from build123d import *

# Parameters (mm, degrees)
CROQUIS2_R              = 5.5
SALIENTE_EXTRUIR1_DEPTH = 18
SALIENTE_EXTRUIR2_DEPTH = 6
CROQUIS4_R              = 3
CORTAR_EXTRUIR1_DEPTH   = 12
CROQUIS5_R              = 1.5
CORTAR_EXTRUIR2_DEPTH   = 6


with BuildPart() as part:
    # Croquis2 → Saliente-Extruir1 (new body)
    with BuildSketch(Plane.XY):
        Circle(CROQUIS2_R)
    extrude(amount=SALIENTE_EXTRUIR1_DEPTH)

    # Croquis3 → Saliente-Extruir2 (add)
    with BuildSketch(Plane(origin=(0, 0, 0), x_dir=(-1, 0, 0), z_dir=(0, 0, -1))):
        Polygon((0, 6.92820323), (-6, 3.464101615), (-6, -3.464101615), (0, -6.92820323), (6, -3.464101615), (6, 3.464101615), align=None)
    extrude(amount=-SALIENTE_EXTRUIR2_DEPTH)

    # Croquis4 → Cortar-Extruir1 (cut)
    with BuildSketch(Plane.XY.offset(18)):
        Circle(CROQUIS4_R)
    extrude(amount=-CORTAR_EXTRUIR1_DEPTH, mode=Mode.SUBTRACT)

    # Croquis5 → Cortar-Extruir2 (cut)
    with BuildSketch(Plane(origin=(0, 0, 0), x_dir=(-1, 0, 0), z_dir=(0, 0, -1))):
        Circle(CROQUIS5_R)
    extrude(amount=-CORTAR_EXTRUIR2_DEPTH, mode=Mode.SUBTRACT)


solid = part.part
The listing builds one solid part. Answer for the finished solid, in the listing's coordinates (mm). A direction names the side the tool comes from. Give positions to 0.01 mm unless a question says otherwise; leave off trailing zeros. Loops run counter-clockwise (first coordinate to the right, second up) from the corner with the lowest first, then second, coordinate; pieces in that order, holes last.
Item 1: A cutting plane is placed at C-C (x = -4.5). Give the vertices of the cut face in (y, z).
Derived:
outline: (-4.33, 0) - (4.33, 0) - (4.33, 6) - (3.16, 6) - (3.16, 18) - (-3.16, 18) - (-3.16, 6) - (-4.33, 6) - close
Item 2: Find the intervals of material crossed by line 1 along Z through (x, y) = (2, 2); line 2 along Y through (x, z) = (0, 13); line 3 along X through (y, z) = (2.75, 8.75), in increasing order.
Derived:
line 1: z = 0 to 6
line 2: y = -5.5 to -3, 3 to 5.5
line 3: x = -4.76 to -1.2, 1.2 to 4.76
Item 3: A tool of negligible diameter and unlimited length cuts with its end or side. For faces 5 (the flat face through (0, -6, 6)), 6 (the flat face through (6, 0, 3)), from which of +Z, -Z, +X, -X, +Y, -Y can it reach the whole face along a straight path? Write none if from no direction.
Derived:
face 5: +Z
face 6: +Z, -Z, +X, +Y, -Y
Item 4: A cutting plane is placed at A-A (z = 3.25). Give the vertices of the cut face in (x, y).
Derived:
outline: (-6, -3.46) - (0, -6.93) - (6, -3.46) - (6, 3.46) - (0, 6.93) - (-6, 3.46) - close; hole circle Ø3 at (0, 0)
Item 5: Each of these flat-tipped pins is pushed along its axis until it touches: pin 1 Ø2.5 at (x, y) = (0, 0) entering from +Z; pin 2 Ø2 at (x, z) = (-3.5, 11.5) entering from +Y. Where does it stop, or does it pass through?
Derived:
pin 1: passes through
pin 2: stops at y = 4.9
Item 6: A cutting plane is placed at D-D (y = -3.25). Give the vertices of the cut face in (x, z), then the cut area to 3 significant figures.
Derived:
outline: (-6, 0) - (6, 0) - (6, 6) - (4.44, 6) - (4.44, 18) - (-4.44, 18) - (-4.44, 6) - (-6, 6) - close
area: 178 mm2
Item 7: Determine the mould class of faces 1 (the flat face through (2.4, -2.4, 18)), 2 (the cylindrical face through (1.5, 0.07, 2.96)), 3 (the flat face through (-2.96, -5.22, 2.96)), 4 (the flat face through (1.3, -1.3, 6)) for opening direction X: +X half, -X half, draft (parallel to the pull), parting line (faces both ways), or undercut.
Derived:
face 1: draft
face 2: undercut
face 3: -X half
face 4: undercut
Item 8: A cutting plane is placed at B-B (y = 0). Give the vertices of the cut face in (x, z).
Derived:
outline: (-6, 0) - (-1.5, 0) - (-1.5, 6) - (-3, 6) - (-3, 18) - (-5.5, 18) - (-5.5, 6) - (-6, 6) - close; (1.5, 0) - (6, 0) - (6, 6) - (5.5, 6) - (5.5, 18) - (3, 18) - (3, 6) - (1.5, 6) - close
